For this review, take the finished solid that the model builds, in its own axes (mm). A direction names the side the tool comes from. Round coordinates to 2 decimals unless told otherwise and drop trailing zeros. Write each loop counter-clockwise with the first axis right and the second up, starting at its lowest first coordinate (ties: lowest second). Pieces come first, ordered by that corner, then holes. Notation, with made-up numbers: (-38, 5) - (20, 5) arc R6 cw to (20, 15) - close; hole circle Ø9 at (-0.75, 35.5). An arc over 180 degrees is marked (long way). Answer in a Markdown table with one row per item. Add a question column.
from build123d import *

# Parameters (mm, degrees)
BOSS_EXTRUDE2_DEPTH     = 40
CUT_EXTRUDE1_DEPTH      = 52.23475383
CUT_EXTRUDE1_DEPTH_BACK = 52.23475383
SKETCH4_R               = 1.5
SKETCH4_W               = 9.017
SKETCH4_H               = 4.572
BOSS_EXTRUDE5_DEPTH     = 3
BOSS_EXTRUDE6_DEPTH     = 10
CUT_EXTRUDE2_DEPTH      = 89.24539648
CUT_EXTRUDE2_DEPTH_BACK = 89.24539648
FILLET3_R               = 10
FILLET4_R               = 1
FILLET5_R               = 2
FILLET6_R               = 1
CUT_EXTRUDE3_DEPTH      = 80.348913103
CUT_EXTRUDE3_DEPTH_BACK = 80.348913103
SKETCH10_R              = 1.75


with BuildPart() as part:
    # Sketch3 → Boss-Extrude2 (new body)
    with BuildSketch(Plane(origin=(0, 0, 0), x_dir=(0, 0, -1), z_dir=(1, 0, 0))):
        Polygon((0, 0), (0, 20), (3.5, 20), (3.5, 3.5), (25, 3.5), (25, 0), align=None)
    extrude(amount=BOSS_EXTRUDE2_DEPTH)

    # Sketch4 → Cut-Extrude1 (cut, two sides: drawn at the far end of the back side and taken through both)
    with BuildSketch(Plane.XY.offset(-CUT_EXTRUDE1_DEPTH_BACK)):
        with Locations(Location((8.3, 13.3, 0), (0, 0, 270))):
            Circle(SKETCH4_R)
        with Locations(Location((31.7, 6.7, 0), (0, 0, 270))):
            Circle(SKETCH4_R)
        with Locations((28.3565, 15.6515)):
            Rectangle(SKETCH4_W, SKETCH4_H)
    extrude(amount=CUT_EXTRUDE1_DEPTH + CUT_EXTRUDE1_DEPTH_BACK, mode=Mode.SUBTRACT)

    # Sketch5 → Boss-Extrude5 (add)
    with BuildSketch(Plane(origin=(40, 0, 0), x_dir=(0, 0, -1), z_dir=(1, 0, 0))):
        Polygon((25, 0), (-24, 0), (-24, 3.5), (-24, 53.5), (3.5, 53.5), (3.5, 3.5), (25, 3.5), align=None)
    extrude(amount=BOSS_EXTRUDE5_DEPTH)

    # Sketch7 → Boss-Extrude6 (add)
    with BuildSketch(Plane(origin=(43, 0, 0), x_dir=(0, 0, -1), z_dir=(1, 0, 0))):
        Polygon((3.5, 3.5), (-21, 3.5), (-21, 0), (25, 0), (25, 3.5), align=None)
        Polygon((-21, 53.5), (-24, 53.5), (-24, 0), (-21, 0), (-21, 3.5), align=None)
    extrude(amount=BOSS_EXTRUDE6_DEPTH)

    # Sketch9 → Cut-Extrude2 (cut, two sides: drawn at the far end of the back side and taken through both)
    with BuildSketch(Plane(origin=(0, 0, 21), x_dir=(-1, 0, 0), z_dir=(0, 0, -1)).offset(-CUT_EXTRUDE2_DEPTH_BACK)):
        with BuildLine():
            Line((-46, 31.5), (-46, 49.5))
            ThreePointArc((-46, 49.5), (-44.5, 51), (-43, 49.5))
            Line((-43, 49.5), (-43, 31.5))
            ThreePointArc((-43, 31.5), (-44.5, 30), (-46, 31.5))
        make_face()
    extrude(amount=CUT_EXTRUDE2_DEPTH + CUT_EXTRUDE2_DEPTH_BACK, mode=Mode.SUBTRACT)

    # Fillet3
    fillet3_edges = [part.edges().sort_by_distance(p)[0] for p in [
        (40, 20, -1.75),
    ]]
    fillet(fillet3_edges, radius=FILLET3_R)

    # Fillet4
    fillet4_edges = [part.edges().sort_by_distance(p)[0] for p in [
        (43, 17.5, 21),
        (43, 51.5, 21),
    ]]
    fillet(fillet4_edges, radius=FILLET4_R)

    # Fillet5
    fillet5_edges = [part.edges().sort_by_distance(p)[0] for p in [
        (40, 15, 0),
        (40, 26.75, 24),
        (43, 28.5, -3.5),
    ]]
    fillet(fillet5_edges, radius=FILLET5_R)

    # Fillet6
    fillet6_edges = [part.edges().sort_by_distance(p)[0] for p in [
        (43.292893219, 3.5, 20.707106781),
        (43, 3.5, 9.25),
        (20.5, 3.5, -3.5),
        (42.414213562, 3.5, -2.914213562),
        (48.5, 3.5, 21),
    ]]
    fillet(fillet6_edges, radius=FILLET6_R)

    # Sketch10 → Cut-Extrude3 (cut, two sides: drawn at the far end of the back side and taken through both)
    with BuildSketch(Plane(origin=(0, 0, 0), x_dir=(-1, 0, 0), z_dir=(0, -1, 0)).offset(-CUT_EXTRUDE3_DEPTH_BACK)):
        with Locations(Location((-44, 12.5, 0), (0, 0, 90))):
            Circle(SKETCH10_R)
        with Locations(Location((-9, 12.5, 0), (0, 0, 90))):
            Circle(SKETCH10_R)
    extrude(amount=CUT_EXTRUDE3_DEPTH + CUT_EXTRUDE3_DEPTH_BACK, mode=Mode.SUBTRACT)


solid = part.part
Q1. Tool access review of faces 1 (the face through (28, 17.938, -2)), 2 (the face through (15, 20, -2)), 3 (the face through (53, 15, 21.4)), 4 (the face through (48, 29, 21)), 5 (the face through (0, 3, -9)): name each direction out of +Z, -Z, +X, -X, +Y, -Y from which nothing blocks a thin tool from reaching the whole face with its end or side.
Q2. Add section C-C on y = 41. State the section outline as (x, z) points, then the cut area to 3 significant figures.
Q3. Add section B-B on z = -12.5. State the section outline as (x, y) points, then the cut area to 3 significant figures.
Q4. To check wall thickness, follow probe 1 along X at (y, z) = (2.65, -12.5); probe 2 along Z at (x, y) = (44, 1.6); probe 3 along X at (y, z) = (13.3, -1.1). State the ranges of each line that lie inside material, in increasing order.
Q5. Add section D-D on x = 21. State the section outline as (y, z) points.
Q6. Draft analysis for pull direction Y (two halves, no side actions). For faces 6 (the face through (32.865, 16, -2)), 7 (the face through (42, 53.5, 14)), 8 (the face through (22, 13, -3.5)), state which applies: released by +Y, released by -Y, zero draft, split by the parting line, or undercut.
Q7. Insertion check: pin 1 Ø13 at (y, z) = (36, 12) entering from -X; pin 2 Ø2.5 at (x, y) = (31.7, 6.7) entering from +Z; pin 3 Ø3.5 at (x, y) = (8.3, 13.3) entering from +Z; pin 4 Ø4.5 at (x, z) = (44, -12.5) entering from +Y. Each pin has a flat end and moves straight along its axis. Give the tip position at first contact, or say it passes through.
Q8. Add section A-A on y = 6.7. State the section outline as (x, z) points, then the cut area to 3 significant figures.
Answer sheet:
| question | item | result |
|---|---|---|
| 1 | face 1 | +Z, -Z |
| 1 | face 2 | +Z, -Z, -X, +Y |
| 1 | face 3 | +Z, -Z, +X, +Y, -Y |
| 1 | face 4 | -Z, +X, +Y |
| 1 | face 5 | +Z, -Z, -X, +Y, -Y |
| 2 | outline | (40, -3.5) - (41, -3.5) arc R2 ccw to (43, -1.5) - (43, 24) - (42, 24) arc R2 ccw to (40, 22) - close; (46, 21) - (53, 21) - (53, 24) - (46, 24) - close |
| 2 | area | 102 mm² |
| 3 | outline | (0, 0) - (7.25, 0) - (7.25, 3.5) - (0, 3.5) - close; (10.75, 0) - (42.25, 0) - (42.25, 3.5) - (10.75, 3.5) - close; (45.75, 0) - (53, 0) - (53, 3.5) - (45.75, 3.5) - close |
| 3 | area | 161 mm² |
| 4 | probe 1 | x = 0 to 7.25, 10.75 to 42.25, 45.75 to 53 |
| 4 | probe 2 | z = -25 to -14.25, -10.75 to 24 |
| 4 | probe 3 | x = 0 to 6.8, 9.8 to 43 |
| 5 | outline | (0, -25) - (3.5, -25) - (3.5, -4.5) arc R1 cw to (4.5, -3.5) - (20, -3.5) - (20, 0) - (0, 0) - close |
| 6 | face 6 | undercut |
| 6 | face 7 | released by +Y |
| 6 | face 8 | zero draft |
| 7 | pin 1 | stops at x = 40 |
| 7 | pin 2 | passes through |
| 7 | pin 3 | stops at z = 0 |
| 7 | pin 4 | stops at y = 3.5 |
| 8 | outline | (0, -3.5) - (30.2, -3.5) - (30.2, 0) - (0, 0) - close; (33.2, -3.5) - (41, -3.5) arc R2 ccw to (43, -1.5) - (43, 20) arc R1 cw to (44, 21) - (53, 21) - (53, 24) - (42, 24) arc R2 ccw to (40, 22) - (40, 2) arc R2 cw to (38, 0) - (33.2, 0) - close |
| 8 | area | 241 mm² |
